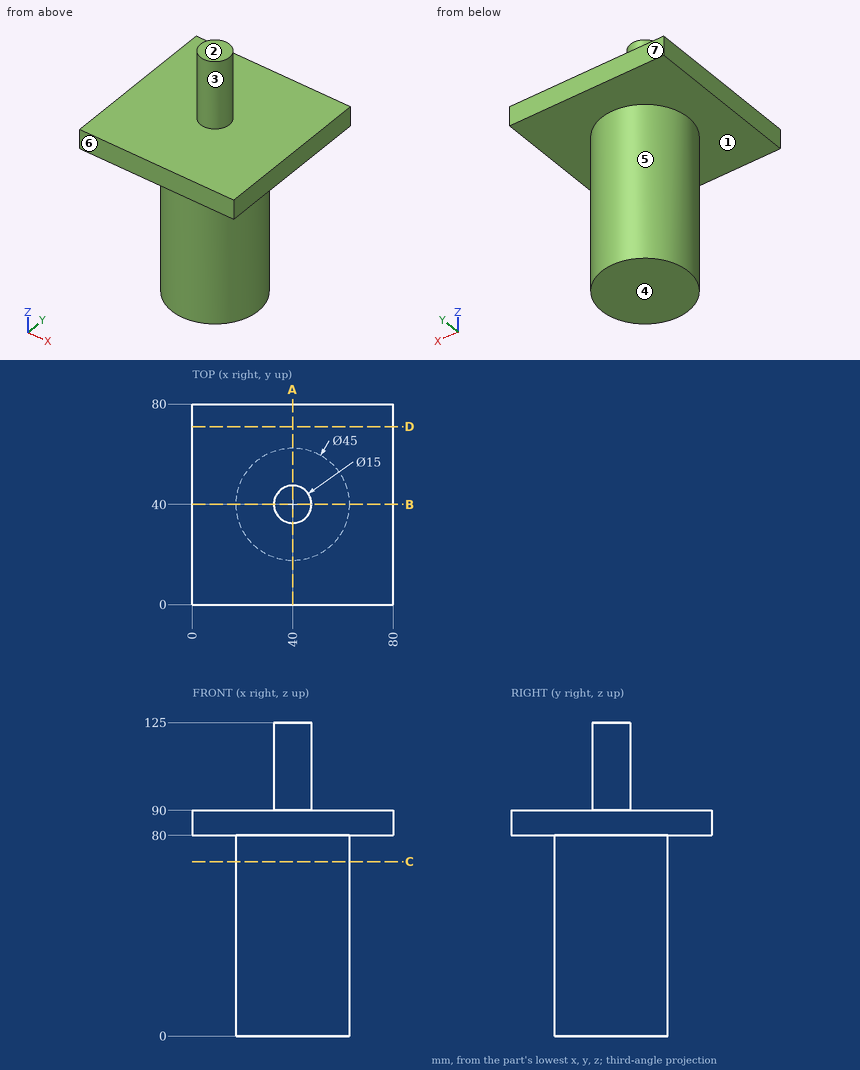
Print and shaded views of the part. All mm, measured from the part's lowest x, y and z. A direction names the side the tool comes from. Give positions to 0.01 mm unless a question says otherwise; leave off trailing zeros. Write each loop counter-clockwise with the first axis right and the second up, starting at its lowest first coordinate (ties: lowest second). Pieces come first, ordered by that corner, then holes. Notation, with made-up numbers: (-33.75, 22) - (-21.75, 22) arc R19 cw to (-21.75, 33) - close; hole circle Ø5 at (51, 49). An arc over 180 degrees is marked (long way). One line per question, with ' | ' between items. Start each with the question number.
(1) Wall check: line 1 along Z through (x, y) = (72, 34); line 2 along Z through (x, y) = (47.5, 31.5); line 3 along Y through (x, z) = (53, 26.5). Give the ranges that are in metal, low to high. Write a range as from..to.
(2) Slice it at C-C on z = 69.5. Write the cut outline in (x, y), plus the area to 3 significant figures.
(3) 3-axis set-ups, long thin cutter, end or side, ignore diameter. For the marked faces 1, 2 and 3: which of +Z, -Z, +X, -X, +Y, -Y reach the whole face in a straight line?
(4) Slice it at A-A on x = 40. Write the cut outline in (y, z), plus the area to 4 significant figures.
(5) Pin check, flat tips, straight feed: P1, Ø4, axis at x = 36, y = 31, coming from the +Z side; P2, Ø12, axis at y = 39.5, z = 96.5, coming from the -X side; P3, Ø5, axis at y = 23, z = 59, coming from the +X side; P4, Ø1.5, axis at x = 10, z = 85.5, coming from the -Y side. Stop position of each tip, or through.
(6) Two-plate mould, pull along Y, no slides. Class the marked faces 4, 5, 6 and 7: +Y half, -Y half, draft (parallel to the pull), parting line (faces both ways), or undercut.
(7) Slice it at D-D on y = 71. Write the cut outline in (x, z).
Results below:
1) line 1: 80..90 | line 2: 0..90 | line 3: 21.64..58.36
2) outline: circle Ø45 at (40, 40) | area: 1,590 mm^2
3) face 1: -Z | face 2: +Z, +X, -X, +Y, -Y | face 3: +Z
4) outline: (0, 80) - (17.5, 80) - (17.5, 0) - (62.5, 0) - (62.5, 80) - (80, 80) - (80, 90) - (47.5, 90) - (47.5, 125) - (32.5, 125) - (32.5, 90) - (0, 90) - close | area: 4,925 mm^2
5) P1: z = 90 | P2: x = 32.5 | P3: x = 57.2 | P4: y = 0
6) face 4: draft | face 5: parting line | face 6: -Y half | face 7: +Y half
7) outline: (0, 80) - (80, 80) - (80, 90) - (0, 90) - close
